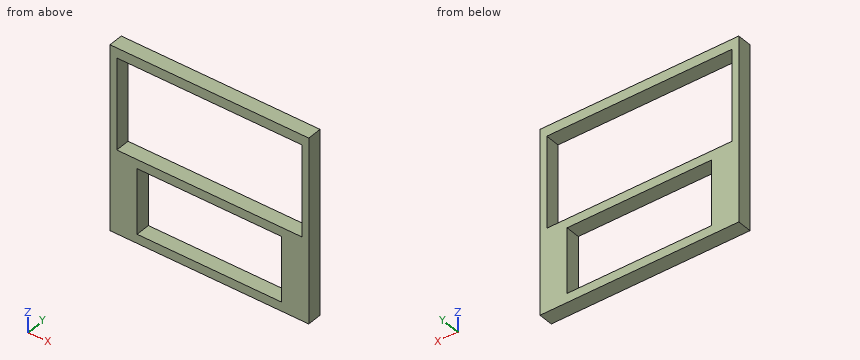
```python
from build123d import *

# Parameters (mm, degrees)
SKETCH1_W           = 110
SKETCH1_H           = 102
SKETCH1_W_2         = 80
SKETCH1_H_2         = 36
BOSS_EXTRUDE1_DEPTH = 8
SKETCH2_W           = 102.5
SKETCH2_H           = 50.5
CUT_EXTRUDE1_DEPTH  = 8


with BuildPart() as part:
    # Sketch1 → Boss-Extrude1 (new body)
    with BuildSketch(Plane(origin=(0, 0, 0), x_dir=(1, 0, 0), z_dir=(0, 1, 0))):
        Rectangle(SKETCH1_W, SKETCH1_H)
        with Locations((0, 28)):
            Rectangle(SKETCH1_W_2, SKETCH1_H_2, mode=Mode.SUBTRACT)
    extrude(amount=BOSS_EXTRUDE1_DEPTH)

    # Sketch2 → Cut-Extrude1 (cut)
    with BuildSketch(Plane(origin=(0, 8, 0), x_dir=(1, 0, 0), z_dir=(0, 1, 0))):
        with Locations((0, -20.25)):
            Rectangle(SKETCH2_W, SKETCH2_H)
    extrude(amount=-CUT_EXTRUDE1_DEPTH, mode=Mode.SUBTRACT)


solid = part.part
```
The model under review builds one solid part; all positions refer to its coordinate system, in mm. Coordinates: 2 decimals unless noted, no trailing zeros. Write each loop counter-clockwise with the first axis right and the second up, starting at its lowest first coordinate (ties: lowest second). Pieces come first, ordered by that corner, then holes. Notation, with made-up numbers: (-35.75, 14.5) - (-22.75, 14.5) arc R7 ccw to (-22.75, 18.5) - close; hole circle Ø9 at (-5, 88.25). An arc over 180 degrees is marked (long way). Answer in a Markdown table with one row per item. Add a question column.
Q1. Consider section A-A on z = 28.5. Give the boundary of the cut face in (x, y).
Q2. Consider section D-D on y = 5. Give the boundary of the cut face in (x, z).
Q3. Clearance check with a flat-ended pin moving along its axis: pin 1 (12 mm diameter, centred on x = -11, z = -19.5, fed in from -Y). State where the tip first meets the part, or that it passes through.
Q4. To check wall thickness, follow line 1 along Z through (x, y) = (21.5, 7.25); line 2 along X through (y, z) = (3, 22.5); line 3 along X through (y, z) = (6.75, -14). State the ranges of each line that lie inside material, in increasing order. Write a range as from..to.
Q5. Consider section C-C on x = 47. Give the boundary of the cut face in (y, z), then the cut area to 3 significant figures.
Q6. Consider section B-B on x = -6. Give the boundary of the cut face in (y, z).
Answers below:
| question | item | result |
|---|---|---|
| 1 | outline | (-55, 0) - (-51.25, 0) - (-51.25, 8) - (-55, 8) - close; (51.25, 0) - (55, 0) - (55, 8) - (51.25, 8) - close |
| 2 | outline | (-55, -51) - (55, -51) - (55, 51) - (-55, 51) - close; hole (-51.25, -5) - (51.25, -5) - (51.25, 45.5) - (-51.25, 45.5) - close; hole (-40, -46) - (40, -46) - (40, -10) - (-40, -10) - close |
| 3 | pin 1 | through |
| 4 | line 1 | -51..-46, -10..-5, 45.5..51 |
| 4 | line 2 | -55..-51.25, 51.25..55 |
| 4 | line 3 | -55..-40, 40..55 |
| 5 | outline | (0, -51) - (8, -51) - (8, -5) - (0, -5) - close; (0, 45.5) - (8, 45.5) - (8, 51) - (0, 51) - close |
| 5 | area | 412 mm² |
| 6 | outline | (0, -51) - (8, -51) - (8, -46) - (0, -46) - close; (0, -10) - (8, -10) - (8, -5) - (0, -5) - close; (0, 45.5) - (8, 45.5) - (8, 51) - (0, 51) - close |
